Input: part model. Units: mm. Frame: model coordinates. Round coordinates to 2 decimals unless told otherwise and drop trailing zeros. Order: outer loops, then holes, each group sorted by start corner. A loop starts at its lowest first (then second) coordinate and runs counter-clockwise, first axis right, second up.
Item 1: Cut plane D-D on y = 0.6. Give the number of separate pieces and of enclosed holes in the cut face, then the cut area to 3 significant figures.
Item 2: Cut plane B-B on z = -30.5. Output: boundary loops of the cut face in (x, y), then the cut area to 3 significant figures.
Item 3: Cut plane A-A on x = 90. Output: boundary loops of the cut face in (y, z), then the cut area to 3 significant figures.
Item 4: Cut plane C-C on x = 26. Output: boundary loops of the cut face in (y, z).
Item 5: Line query: L1, parallel to X at y = 3.05, z = -40; L2, parallel to Z at x = 90, y = 0.9; L3, parallel to X at y = 2.95, z = -19. Output: solid intervals per line, ascending.
Item 6: First-contact query: pin 1 (19.5 mm diameter, centred on x = 90, z = -20, fed in from +Y); pin 2 (1 mm diameter, centred on y = 1.5, z = -69, fed in from +X). Flat tips, straight axial feed; report the tip coordinate or a pass-through.
```python
from build123d import *

# Parameters (mm, degrees)
ESQUISSE1_W                         = 180
ESQUISSE1_H                         = 80
BOSS_EXTRU_1_DEPTH                  = 4
ENL_V_MAT_EXTRU_1_DEPTH             = 4
ENL_V_MAT_EXTRU_2_DEPTH             = 4
ENL_V_MAT_EXTRU_5_REACH             = 6
ESQUISSE11_W                        = 12
ESQUISSE11_H                        = 40
ENL_V_MAT_EXTRU_5_DIRECTION_2_DEPTH = 1
ENL_V_MAT_EXTRU_6_REACH             = 6
ESQUISSE14_R                        = 7.5


with BuildPart() as part:
    # Esquisse1 → Boss.-Extru.1 (new body)
    with BuildSketch(Plane(origin=(0, 0, 0), x_dir=(1, 0, 0), z_dir=(0, 1, 0))):
        with Locations((90, 40)):
            Rectangle(ESQUISSE1_W, ESQUISSE1_H)
    extrude(amount=BOSS_EXTRU_1_DEPTH)

    # Esquisse2 → Enlèv. mat.-Extru.1 (cut)
    with BuildSketch(Plane(origin=(0, 4, 0), x_dir=(1, 0, 0), z_dir=(0, 1, 0))):
        Polygon((30, 0), (0, 15), (0, 0), align=None)
        Polygon((30, 80), (0, 65), (0, 80), align=None)
        Polygon((150, 0), (180, 15), (180, 0), align=None)
        Polygon((150, 80), (180, 80), (180, 65), align=None)
    extrude(amount=-ENL_V_MAT_EXTRU_1_DEPTH, mode=Mode.SUBTRACT)

    # Esquisse3 → Enlèv. mat.-Extru.2 (cut)
    with BuildSketch(Plane(origin=(0, 4, 0), x_dir=(1, 0, 0), z_dir=(0, 1, 0))):
        with BuildLine():
            Line((65.05, 38), (65.05, 18))
            ThreePointArc((65.05, 18), (64, 16.95), (62.95, 18))
            Line((62.95, 18), (62.95, 38))
            ThreePointArc((62.95, 38), (64, 39.05), (65.05, 38))
        make_face()
        with BuildLine():
            Line((50.95, 18), (50.95, 38))
            ThreePointArc((50.95, 38), (52, 39.05), (53.05, 38))
            Line((53.05, 38), (53.05, 18))
            ThreePointArc((53.05, 18), (52, 16.95), (50.95, 18))
        make_face()
        with BuildLine():
            Line((129.05, 18), (129.05, 38))
            ThreePointArc((129.05, 38), (128, 39.05), (126.95, 38))
            Line((126.95, 38), (126.95, 18))
            ThreePointArc((126.95, 18), (128, 16.95), (129.05, 18))
        make_face()
        with BuildLine():
            Line((114.95, 38), (114.95, 18))
            ThreePointArc((114.95, 18), (116, 16.95), (117.05, 18))
            Line((117.05, 18), (117.05, 38))
            ThreePointArc((117.05, 38), (116, 39.05), (114.95, 38))
        make_face()
        with BuildLine():
            Line((50.95, 62), (50.95, 42))
            ThreePointArc((50.95, 42), (52, 40.95), (53.05, 42))
            Line((53.05, 42), (53.05, 62))
            ThreePointArc((53.05, 62), (52, 63.05), (50.95, 62))
        make_face()
        with BuildLine():
            Line((65.05, 42), (65.05, 62))
            ThreePointArc((65.05, 62), (64, 63.05), (62.95, 62))
            Line((62.95, 62), (62.95, 42))
            ThreePointArc((62.95, 42), (64, 40.95), (65.05, 42))
        make_face()
        with BuildLine():
            Line((114.95, 42), (114.95, 62))
            ThreePointArc((114.95, 62), (116, 63.05), (117.05, 62))
            Line((117.05, 62), (117.05, 42))
            ThreePointArc((117.05, 42), (116, 40.95), (114.95, 42))
        make_face()
        with BuildLine():
            Line((129.05, 62), (129.05, 42))
            ThreePointArc((129.05, 42), (128, 40.95), (126.95, 42))
            Line((126.95, 42), (126.95, 62))
            ThreePointArc((126.95, 62), (128, 63.05), (129.05, 62))
        make_face()
    extrude(amount=-ENL_V_MAT_EXTRU_2_DEPTH, mode=Mode.SUBTRACT)

    # Esquisse11 → Enlèv. mat.-Extru.5 (cut, up to next)
    with BuildSketch(Plane(origin=(0, 4, 0), x_dir=(1, 0, 0), z_dir=(0, 1, 0)), mode=Mode.PRIVATE) as enl_v_mat_extru_5_sk1:
        with Locations((34, 40)):
            Rectangle(ESQUISSE11_W, ESQUISSE11_H)
    enl_v_mat_extru_5_tool1 = extrude(enl_v_mat_extru_5_sk1.sketch, amount=-ENL_V_MAT_EXTRU_5_REACH, mode=Mode.PRIVATE) & part.part
    add(enl_v_mat_extru_5_tool1.solids().sort_by_distance((34, 4, -40))[0], mode=Mode.SUBTRACT)
    # Esquisse11 → Enlèv. mat.-Extru.5 (cut, up to next)
    with BuildSketch(Plane(origin=(0, 4, 0), x_dir=(1, 0, 0), z_dir=(0, 1, 0)), mode=Mode.PRIVATE) as enl_v_mat_extru_5_sk2:
        with Locations((146, 40)):
            Rectangle(ESQUISSE11_W, ESQUISSE11_H)
    enl_v_mat_extru_5_tool2 = extrude(enl_v_mat_extru_5_sk2.sketch, amount=-ENL_V_MAT_EXTRU_5_REACH, mode=Mode.PRIVATE) & part.part
    add(enl_v_mat_extru_5_tool2.solids().sort_by_distance((146, 4, -40))[0], mode=Mode.SUBTRACT)

    # Esquisse11 → Enlèv. mat.-Extru.5 direction 2 (cut)
    with BuildSketch(Plane(origin=(0, 4, 0), x_dir=(1, 0, 0), z_dir=(0, 1, 0))):
        with Locations((34, 40)):
            Rectangle(ESQUISSE11_W, ESQUISSE11_H)
        with Locations((146, 40)):
            Rectangle(ESQUISSE11_W, ESQUISSE11_H)
    extrude(amount=ENL_V_MAT_EXTRU_5_DIRECTION_2_DEPTH, mode=Mode.SUBTRACT)

    # Esquisse14 → Enlèv. mat.-Extru.6 (cut, up to next)
    with BuildSketch(Plane(origin=(0, 4, 0), x_dir=(1, 0, 0), z_dir=(0, 1, 0)), mode=Mode.PRIVATE) as enl_v_mat_extru_6_sk1:
        with Locations((90, 60)):
            Circle(ESQUISSE14_R)
    enl_v_mat_extru_6_tool1 = extrude(enl_v_mat_extru_6_sk1.sketch, amount=-ENL_V_MAT_EXTRU_6_REACH, mode=Mode.PRIVATE) & part.part
    add(enl_v_mat_extru_6_tool1.solids().sort_by_distance((90, 4, -60))[0], mode=Mode.SUBTRACT)
    # Esquisse14 → Enlèv. mat.-Extru.6 (cut, up to next)
    with BuildSketch(Plane(origin=(0, 4, 0), x_dir=(1, 0, 0), z_dir=(0, 1, 0)), mode=Mode.PRIVATE) as enl_v_mat_extru_6_sk2:
        with Locations((90, 40)):
            Circle(ESQUISSE14_R)
    enl_v_mat_extru_6_tool2 = extrude(enl_v_mat_extru_6_sk2.sketch, amount=-ENL_V_MAT_EXTRU_6_REACH, mode=Mode.PRIVATE) & part.part
    add(enl_v_mat_extru_6_tool2.solids().sort_by_distance((90, 4, -40))[0], mode=Mode.SUBTRACT)
    # Esquisse14 → Enlèv. mat.-Extru.6 (cut, up to next)
    with BuildSketch(Plane(origin=(0, 4, 0), x_dir=(1, 0, 0), z_dir=(0, 1, 0)), mode=Mode.PRIVATE) as enl_v_mat_extru_6_sk3:
        with Locations((90, 20)):
            Circle(ESQUISSE14_R)
    enl_v_mat_extru_6_tool3 = extrude(enl_v_mat_extru_6_sk3.sketch, amount=-ENL_V_MAT_EXTRU_6_REACH, mode=Mode.PRIVATE) & part.part
    add(enl_v_mat_extru_6_tool3.solids().sort_by_distance((90, 4, -20))[0], mode=Mode.SUBTRACT)


solid = part.part
```
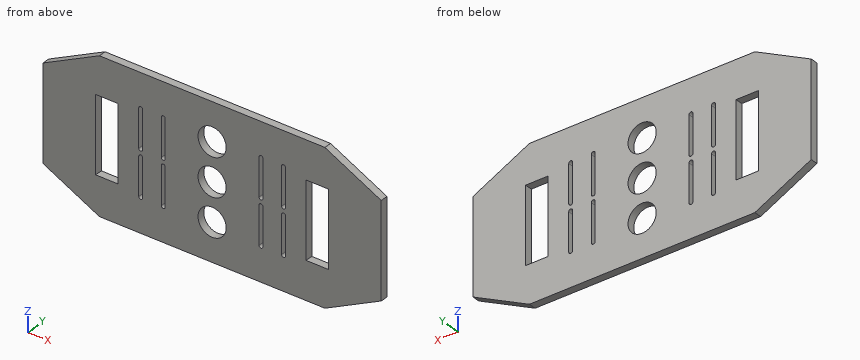
From the geometry:
1. separate pieces: 1
1. enclosed holes: 13
1. area: 11,600 mm2
2. outline: (0, 0) - (28, 0) - (28, 4) - (0, 4) - close; (40, 0) - (50.95, 0) - (50.95, 4) - (40, 4) - close; (53.05, 0) - (62.95, 0) - (62.95, 4) - (53.05, 4) - close; (65.05, 0) - (114.95, 0) - (114.95, 4) - (65.05, 4) - close; (117.05, 0) - (126.95, 0) - (126.95, 4) - (117.05, 4) - close; (129.05, 0) - (140, 0) - (140, 4) - (129.05, 4) - close; (152, 0) - (180, 0) - (180, 4) - (152, 4) - close
2. area: 590 mm2
3. outline: (0, -80) - (4, -80) - (4, -67.5) - (0, -67.5) - close; (0, -52.5) - (4, -52.5) - (4, -47.5) - (0, -47.5) - close; (0, -32.5) - (4, -32.5) - (4, -27.5) - (0, -27.5) - close; (0, -12.5) - (4, -12.5) - (4, 0) - (0, 0) - close
3. area: 140 mm2
4. outline: (0, -78) - (4, -78) - (4, -2) - (0, -2) - close
5. L1: x = 0 to 28, 40 to 82.5, 97.5 to 140, 152 to 180
5. L2: z = -80 to -67.5, -52.5 to -47.5, -32.5 to -27.5, -12.5 to 0
5. L3: x = 0 to 50.95, 53.05 to 62.95, 65.05 to 82.57, 97.43 to 114.95, 117.05 to 126.95, 129.05 to 180
6. pin 1: stops at y = 4
6. pin 2: stops at x = 173
